Job drawing, mm, ordinate dimensions from the low corner. One solid piece. A direction names the side the tool comes from. Round coordinates to 2 decimals unless told otherwise and drop trailing zeros. Write each loop counter-clockwise with the first axis right and the second up, starting at its lowest first coordinate (ties: lowest second). Pieces come first, ordered by that corner, then holes.
1) Drill centre lines: L1, parallel to Z at x = 12.7, y = 12.05 (1 decimal); L2, parallel to Z at x = 12.7, y = 3.25; L3, parallel to Z at x = 11.75, y = 14.25 (1 decimal). Where is each one in solid material? Low to high.
2) Saw through at C-C on x = 5.75. Write the cut outline in (y, z).
3) Which spindle directions (+Z, -Z, +X, -X, +Y, -Y) get a long thin tool onto all of the face, cutting with end or side? Do the marked faces 1 and 2. Say none if no direction does.
4) Flat gauge pins, fed straight in: pin 1 (1.5 mm diameter, centred on y = 8.5, z = 22, fed in from +X); pin 2 (8 mm diameter, centred on x = 19, y = 5, fed in from -Z); pin 3 (4 mm diameter, centred on y = 8.5, z = 5, fed in from +X); pin 4 (3 mm diameter, centred on x = 7, y = 12.5, fed in from +Z) (1 decimal). Where does each tip first touch, or does it go through?
5) Saw through at A-A on x = 12.7. Count the separate pieces of the cut face and the enclosed holes in it, and give its area (3 significant figures).
6) Pull direction Z, two halves, no side cores. Call the marked faces 3, 4 and 5: +Z half, -Z half, draft (parallel to the pull), parting line (faces both ways), or undercut.
7) Saw through at B-B on z = 12.7. Write the cut outline in (x, y), and give its area (3 significant figures).
8) Saw through at D-D on y = 11.25. Write the cut outline in (x, z) (1 decimal).
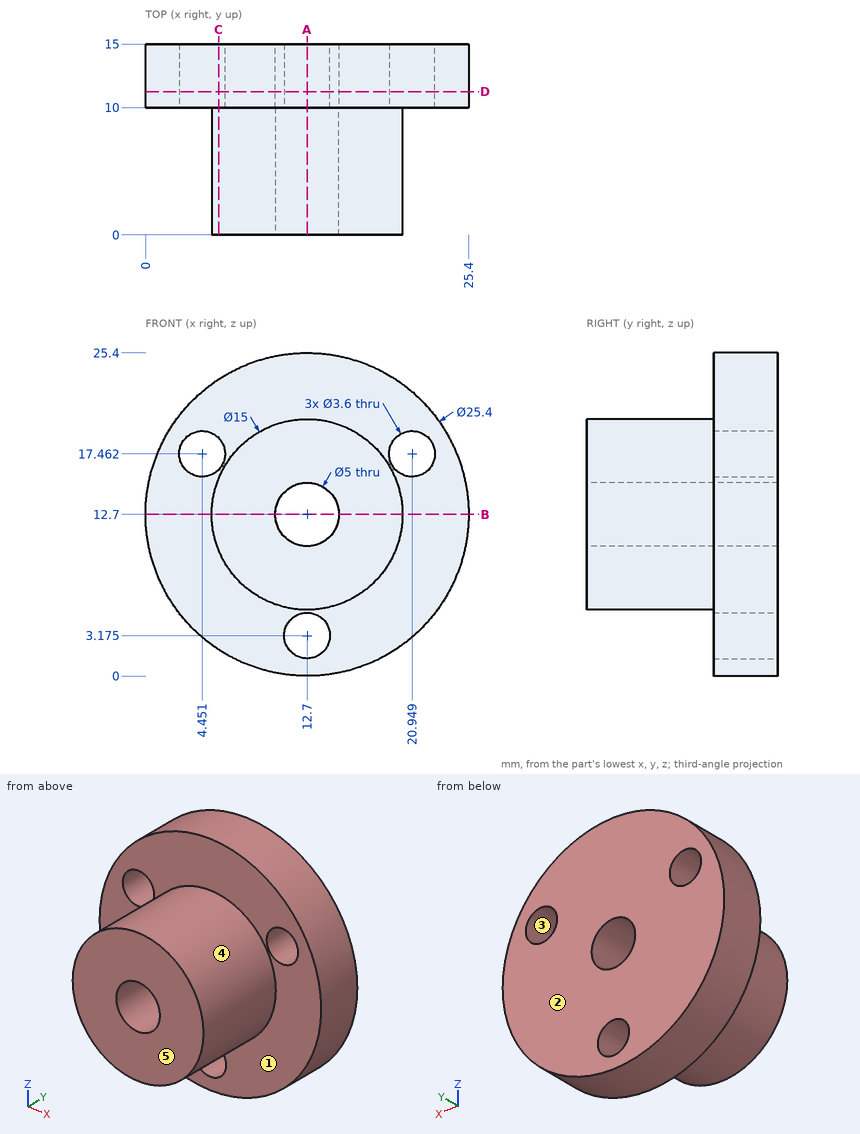
Completed:
1. L1: z = 0 to 1.4, 5 to 10.2, 15.2 to 25.4
1. L2: z = 5.2 to 10.2, 15.2 to 20.2
1. L3: z = 0 to 1.6, 4.7 to 10.4, 15 to 25.4
2. outline: (0, 9.88) - (10, 9.88) - (10, 2.07) - (15, 2.07) - (15, 16.22) - (10, 16.22) - (10, 15.52) - (0, 15.52) - close; (10, 18.71) - (15, 18.71) - (15, 23.33) - (10, 23.33) - close
3. face 1: -Y
3. face 2: +Z, -Z, +X, -X, +Y
4. pin 1: passes through
4. pin 2: stops at z = 5.56
4. pin 3: stops at x = 23.68
4. pin 4: stops at z = 24.7
5. separate pieces: 3
5. enclosed holes: 0
5. area: 184 mm2
6. face 3: undercut
6. face 4: parting line
6. face 5: draft
7. outline: (0, 10) - (5.2, 10) - (5.2, 0) - (10.2, 0) - (10.2, 15) - (0, 15) - close; (15.2, 0) - (20.2, 0) - (20.2, 10) - (25.4, 10) - (25.4, 15) - (15.2, 15) - close
7. area: 202 mm2
8. outline: circle Ø25.4 at (12.7, 12.7); hole circle Ø3.6 at (4.5, 17.5); hole circle Ø5 at (12.7, 12.7); hole circle Ø3.6 at (12.7, 3.2); hole circle Ø3.6 at (20.9, 17.5)
